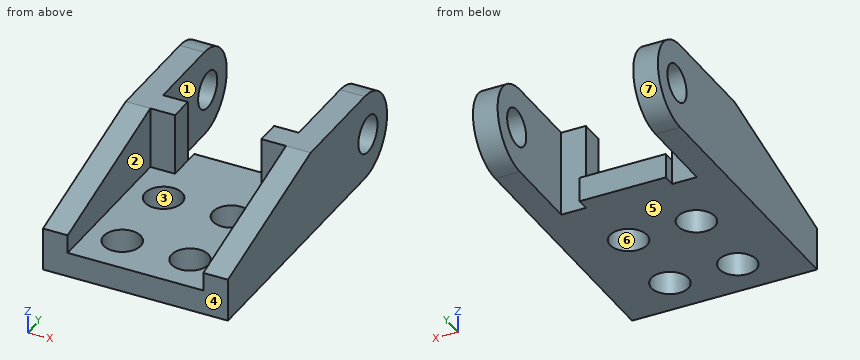
from build123d import *

# Parameters (mm, degrees)
SKETCH_1_W          = 15
SKETCH_1_H          = 25
EXTRUDE_1_DEPTH     = 7
CUT_EXTRUDE_1_DEPTH = 5
SKETCH_3_W          = 2
SKETCH_3_H          = 10
CUT_EXTRUDE_2_DEPTH = 13
SKETCH_4_W          = 2
SKETCH_4_H          = 3
CUT_EXTRUDE_3_DEPTH = 20.345542122
SKETCH_5_W          = 7
SKETCH_5_H          = 6
CUT_EXTRUDE_4_DEPTH = 13
SKETCH_6_R          = 1.5
EXTRUDE_2_DEPTH     = 2
EXTRUDE_START       = 2
SKETCH_7_R          = 1.5
EXTRUDE_3_DEPTH     = 2
CUT_EXTRUDE_5_DEPTH = 21.742468513
SKETCH_9_R          = 1.5
CUT_EXTRUDE_6_DEPTH = 16.411035007
SKETCH_10_W         = 4
SKETCH_10_H         = 10
EXTRUDE_5_DEPTH     = 7
SKETCH_12_W         = 2
SKETCH_12_H         = 10
CUT_EXTRUDE_7_DEPTH = 17.170961629
SKETCH_14_R         = 1.5
CUT_EXTRUDE_9_DEPTH = 21.742468513
FILLET_1_RADIUS     = 3.5
FILLET_1_LENGTH     = 2
FILLET_2_RADIUS     = 3.5
FILLET_2_LENGTH     = 2


with BuildPart() as part:
    # Эскиз1 → Бобышка-Вытянуть1 (new body)
    with BuildSketch(Plane.XY):
        Rectangle(SKETCH_1_W, SKETCH_1_H)
    extrude(amount=EXTRUDE_1_DEPTH)

    # Эскиз2 → Вырез-Вытянуть1 (cut)
    with BuildSketch(Plane.XY.offset(7)):
        Polygon((-3.5, 0.5), (-5.5, 0.5), (-5.5, -12.5), (5.5, -12.5), (5.5, 0.5), (3.5, 0.5), (3.5, 12.5), (-3.5, 12.5), align=None)
    extrude(amount=-CUT_EXTRUDE_1_DEPTH, mode=Mode.SUBTRACT)

    # Эскиз3 → Вырез-Вытянуть2 (cut)
    with BuildSketch(Plane.XY.offset(7)):
        with Locations((-6.5, 7.5)):
            Rectangle(SKETCH_3_W, SKETCH_3_H)
        with Locations((6.5, 7.5)):
            Rectangle(SKETCH_3_W, SKETCH_3_H)
    extrude(amount=-CUT_EXTRUDE_2_DEPTH, mode=Mode.SUBTRACT)

    # Эскиз4 → Вырез-Вытянуть3 (cut, through all)
    with BuildSketch(Plane.ZY.offset(5.5)):
        with Locations((6, 11)):
            Rectangle(SKETCH_4_W, SKETCH_4_H)
        with Locations((1, 11)):
            Rectangle(SKETCH_4_W, SKETCH_4_H)
    extrude(amount=-CUT_EXTRUDE_3_DEPTH, mode=Mode.SUBTRACT)

    # Эскиз5 → Вырез-Вытянуть4 (cut)
    with BuildSketch(Plane.XY.offset(2)):
        with Locations((0, 6.5)):
            Rectangle(SKETCH_5_W, SKETCH_5_H)
    extrude(amount=-CUT_EXTRUDE_4_DEPTH, mode=Mode.SUBTRACT)

    # Эскиз6 → Бобышка-Вытянуть2 (add)
    with BuildSketch(Plane.ZY.offset(5.5)):
        with Locations(Location((3.5, 9.5, 0), (0, 0, 180))):
            Circle(SKETCH_6_R)
    extrude(amount=EXTRUDE_2_DEPTH)

    # Эскиз7 → Бобышка-Вытянуть3 (add)
    with BuildSketch(Plane(origin=(5.5, 0, 0), x_dir=(0, 0, -1), z_dir=(1, 0, 0)).offset(EXTRUDE_START)):
        with Locations((-3.5, 9.5)):
            Circle(SKETCH_7_R)
    extrude(amount=-EXTRUDE_3_DEPTH)

    # Эскиз8 → Вырез-Вытянуть5 (cut, through all)
    with BuildSketch(Plane.ZY.offset(7.5)):
        Polygon((7, 0.5), (3.5, -12.5), (7, -12.5), align=None)
    extrude(amount=-CUT_EXTRUDE_5_DEPTH, mode=Mode.SUBTRACT)

    # Эскиз9 → Вырез-Вытянуть6 (cut, through all)
    with BuildSketch(Plane.XY.offset(2)):
        with Locations((-2.75, -2.75)):
            Circle(SKETCH_9_R)
        with Locations((2.75, -2.75)):
            Circle(SKETCH_9_R)
        with Locations((-2.75, -9.25)):
            Circle(SKETCH_9_R)
        with Locations((2.75, -9.25)):
            Circle(SKETCH_9_R)
    extrude(amount=-CUT_EXTRUDE_6_DEPTH, mode=Mode.SUBTRACT)

    # Эскиз10 → Бобышка-Вытянуть5 (add)
    with BuildSketch(Plane.XY.offset(7)):
        with Locations((-5.5, 7.5)):
            Rectangle(SKETCH_10_W, SKETCH_10_H)
        with Locations((5.5, 7.5)):
            Rectangle(SKETCH_10_W, SKETCH_10_H)
    extrude(amount=-EXTRUDE_5_DEPTH)

    # Эскиз12 → Вырез-Вытянуть7 (cut, through all)
    with BuildSketch(Plane.XY.offset(7)):
        with Locations((4.5, 7.5)):
            Rectangle(SKETCH_12_W, SKETCH_12_H)
        with Locations((-4.5, 7.5)):
            Rectangle(SKETCH_12_W, SKETCH_12_H)
    extrude(amount=-CUT_EXTRUDE_7_DEPTH, mode=Mode.SUBTRACT)

    # Эскиз14 → Вырез-Вытянуть9 (cut, through all)
    with BuildSketch(Plane.ZY.offset(7.5)):
        with Locations(Location((3.5, 9.5, 0), (0, 0, 270))):
            Circle(SKETCH_14_R)
    extrude(amount=-CUT_EXTRUDE_9_DEPTH, mode=Mode.SUBTRACT)

    # Скругление1: full round fillet: the end face becomes a half cylinder, R = half its width
    fillet_1_face = Plane((-6.5, 12.5, 3.5), x_dir=(1, 0, 0), z_dir=(0, 1, 0))  # on the end face: x along it, z out of the body
    fillet_1_slab = fillet_1_face.offset(-FILLET_1_RADIUS / 2) * Box(FILLET_1_LENGTH, 2 * FILLET_1_RADIUS, FILLET_1_RADIUS, mode=Mode.PRIVATE)  # the body's end, R deep
    fillet_1_round = Plane((-6.5, 9, 3.5), x_dir=(0, 1, 0), z_dir=(1, 0, 0)) * Cylinder(FILLET_1_RADIUS, FILLET_1_LENGTH, mode=Mode.PRIVATE)  # its axis R under the face
    add(fillet_1_slab - fillet_1_round, mode=Mode.SUBTRACT)

    # Скругление2: full round fillet: the end face becomes a half cylinder, R = half its width
    fillet_2_face = Plane((6.5, 12.5, 3.5), x_dir=(1, 0, 0), z_dir=(0, 1, 0))  # on the end face: x along it, z out of the body
    fillet_2_slab = fillet_2_face.offset(-FILLET_2_RADIUS / 2) * Box(FILLET_2_LENGTH, 2 * FILLET_2_RADIUS, FILLET_2_RADIUS, mode=Mode.PRIVATE)  # the body's end, R deep
    fillet_2_round = Plane((6.5, 9, 3.5), x_dir=(0, 1, 0), z_dir=(1, 0, 0)) * Cylinder(FILLET_2_RADIUS, FILLET_2_LENGTH, mode=Mode.PRIVATE)  # its axis R under the face
    add(fillet_2_slab - fillet_2_round, mode=Mode.SUBTRACT)


solid = part.part
Here's how the part is built. I have some questions about the finished solid (model axes, mm). Face numbers are marked on the shaded views. A direction names the side the tool comes from. Coordinates: 2 decimals unless noted, no trailing zeros. Write each loop counter-clockwise with the first axis right and the second up, starting at its lowest first coordinate (ties: lowest second). Pieces come first, ordered by that corner, then holes. Notation, with made-up numbers: (5, 35) - (35, 35) arc R5 ccw to (35, 44) - close; hole circle Ø4 at (-19, 19). An arc over 180 degrees is marked (long way). Use one line per item in the form item = value.
1) Suppose I cut it at A-A, the plane x = -2.75. Write out the boundary of the cut face in (y, z), plus the area to 3 significant figures.
Solved:
outline = (-12.5, 0) - (-10.75, 0) - (-10.75, 2) - (-12.5, 2) - close; (-7.75, 0) - (-4.25, 0) - (-4.25, 2) - (-7.75, 2) - close; (-1.25, 0) - (3.5, 0) - (3.5, 2) - (-1.25, 2) - close
area = 20.0 mm2
2) Suppose I cut it at C-C, the plane x = 6. Write out the boundary of the cut face in (y, z), plus the area to 3 significant figures.
Solved:
outline = (-12.5, 0) - (9, 0) arc R3.5 ccw to (9, 7) - (0.5, 7) - (-12.5, 3.5) - close; hole circle Ø3 at (9.5, 3.5)
area = 140 mm2
3) Suppose I cut it at D-D, the plane z = 5.5. Write out the boundary of the cut face in (x, y).
Solved:
outline = (-7.5, -5.07) - (-5.5, -5.07) - (-5.5, 0.5) - (-3.5, 0.5) - (-3.5, 2.5) - (-5.5, 2.5) - (-5.5, 11.87) - (-7.5, 11.87) - close; (3.5, 0.5) - (5.5, 0.5) - (5.5, -5.07) - (7.5, -5.07) - (7.5, 11.87) - (5.5, 11.87) - (5.5, 2.5) - (3.5, 2.5) - close
4) I need wall thicknesses on line 1 (Y direction, x = 2.75, z = 0.45); line 2 (X direction, y = 6.25, z = 6.5); line 3 (Z direction, x = -3.25, y = -11). Which ranges of each line are inside material? Lowest first, please.
Solved:
line_1 = -12.5 to -10.75, -7.75 to -4.25, -1.25 to 3.5
line_2 = -7.5 to -5.5, 5.5 to 7.5
line_3 = 0 to 2
5) Suppose I cut it at B-B, the plane y = 6. Write out the boundary of the cut face in (x, z), plus the area to 3 significant figures.
Solved:
outline = (-7.5, 0) - (-5.5, 0) - (-5.5, 7) - (-7.5, 7) - close; (5.5, 0) - (7.5, 0) - (7.5, 7) - (5.5, 7) - close
area = 28.0 mm2
6) Thinking about a two-plate mould opening in Y: for the marked faces 4, 5, 6 and 7, which applies, released by +Y, released by -Y, zero draft, split by the parting line, or undercut?
Solved:
face_4 = released by -Y
face_5 = zero draft
face_6 = undercut
face_7 = released by +Y
7) I'm going to push flat-ended pins straight in: P1, Ø1, axis at y = -8.5, z = 5.5, coming from the +X side; P2, Ø1, axis at x = 0.5, y = -0.5, coming from the +Z side; P3, Ø6, axis at x = 5, y = -3, coming from the +Z side; P4, Ø4, axis at y = -6.5, z = 6, coming from the +X side. Where does each tip first touch, or does it pass through?
Solved:
P1 = through
P2 = 2
P3 = 6.85
P4 = 7.5
8) On a 3-axis mill with a long thin cutter (end or side, diameter ignored), from which of +Z, -Z, +X, -X, +Y, -Y can I reach the whole of each face in a straight line? I mean the marked faces 1, 2 and 3. Say none if no direction works.
Solved:
face_1 = +Z, -Z, +Y
face_2 = +Z, -Y
face_3 = +Z, -Z
